Work out the finished part from the listing and answer in its coordinate system (mm). A direction names the side the tool comes from. Coordinates: 2 decimals unless noted, no trailing zeros. Loops run counter-clockwise (first coordinate to the right, second up) from the corner with the lowest first, then second, coordinate; pieces in that order, holes last.
```python
from build123d import *

# Parameters (mm, degrees)
SALIENTE_EXTRUIR1_DEPTH    = 10.8
CORTAR_EXTRUIR1_DEPTH      = 28.076558127
CORTAR_EXTRUIR1_DEPTH_BACK = 28.076558127
CROQUIS4_W                 = 1.025
CROQUIS4_H                 = 17.1
CORTAR_EXTRUIR2_DEPTH      = 33.246404838
CORTAR_EXTRUIR2_DEPTH_BACK = 5.4
CROQUIS5_R                 = 3


with BuildPart() as part:
    # Croquis2 → Saliente-Extruir1 (new, symmetric)
    with BuildSketch(Plane(origin=(0, 0, 0), x_dir=(0, 0, -1), z_dir=(1, 0, 0))):
        with BuildLine():
            Line((11.7, 11.4), (11.7, -21.9))
            Line((11.7, -21.9), (-11.7, -21.9))
            Line((-11.7, -21.9), (-11.7, -12))
            Line((-11.7, -12), (-5.1, -12))
            Line((-5.1, -12), (-5.1, 3))
            ThreePointArc((-5.1, 3), (-3.495742753, 20.791485505), (11.7, 11.4))
        make_face()
    extrude(amount=SALIENTE_EXTRUIR1_DEPTH, both=True)

    # Croquis4 → Cortar-Extruir1 (cut, two sides: drawn at the far end of the back side and taken through both)
    with BuildSketch(Plane.XY.offset(-CORTAR_EXTRUIR1_DEPTH_BACK)):
        with Locations((-10.2875, 13.35)):
            Rectangle(CROQUIS4_W, CROQUIS4_H)
    extrude(amount=CORTAR_EXTRUIR1_DEPTH + CORTAR_EXTRUIR1_DEPTH_BACK, mode=Mode.SUBTRACT)

    # Croquis5 → Cortar-Extruir2 (cut, two sides: drawn at the far end of the back side and taken through both)
    with BuildSketch(Plane.ZY.offset(9.775).offset(-CORTAR_EXTRUIR2_DEPTH_BACK)):
        with Locations(Location((0, 13.35, 0), (0, 0, 90))):
            Circle(CROQUIS5_R)
    extrude(amount=CORTAR_EXTRUIR2_DEPTH + CORTAR_EXTRUIR2_DEPTH_BACK, mode=Mode.SUBTRACT)


solid = part.part
```
1. A cutting plane is placed at B-B, the plane y = 13.35. Give the vertices of the cut face in (x, z) (3 decimals), then the cut area to 3 significant figures.
2. A cutting plane is placed at D-D, the plane y = -5. Give the vertices of the cut face in (x, z), then the cut area to 3 significant figures.
3. A cutting plane is placed at C-C, the plane x = 7.75. Give the vertices of the cut face in (y, z).
4. For faces 5 (the cylindrical face through (0.151, 20.654, 3.761)), 6 (the flat face through (-9.775, 13, -4)), 7 (the flat face through (0, -12, 8)), determine the directions among +Z, -Z, +X, -X, +Y, -Y from which every point of the face is accessible in a straight line to the end or side of a thin tool.
5. Straight lines are drawn through the part: probe 1 along X at (y, z) = (16, -0.75) (3 decimals); probe 2 along Z at (x, y) = (-6, 13.35); probe 3 along Z at (x, y) = (-8.25, 15). For each, find the intervals that lie inside material, in ascending order.
6. A cutting plane is placed at A-A, the plane z = -1.2. Give the vertices of the cut face in (x, y) (3 decimals), then the cut area to 3 significant figures.
7. Determine the mould class of faces 1 (the flat face through (0, -5, 5.1)), 2 (the cylindrical face through (-7.037, 10.353, -0.132)), 3 (the flat face through (-10, 4.8, -2)), 4 (the flat face through (-4.375, 13, 0)) for opening direction Z: released by +Z, released by -Z, zero draft, split by the parting line, or undercut.
8. Each of these flat-tipped pins is pushed along its axis until it touches: P1, Ø1.5, axis at x = -4.5, y = 7, coming from the +Z side; P2, Ø5, axis at x = 0.5, y = -7.5, coming from the +Z side; P3, Ø12, axis at x = -2.5, y = -2, coming from the +Z side. Where does it stop, or does it pass through?
Answers below:
1. outline: (-9.775, -11.517) - (10.8, -11.517) - (10.8, 9.117) - (-9.775, 9.117) - (-9.775, 3) - (-4.375, 3) - (-4.375, -3) - (-9.775, -3) - close
1. area: 392 mm2
2. outline: (-10.8, -11.7) - (10.8, -11.7) - (10.8, 5.1) - (-10.8, 5.1) - close
2. area: 363 mm2
3. outline: (-21.9, -11.7) - (11.4, -11.7) arc R10.5 ccw (long way) to (3, 5.1) - (-12, 5.1) - (-12, 11.7) - (-21.9, 11.7) - close
4. face 5: +X, -X
4. face 6: +Z, -Z, -X, +Y
4. face 7: +Z, +X, -X
5. probe 1: x = -4.375 to 10.8
5. probe 2: z = -11.52 to -3, 3 to 9.12
5. probe 3: z = -11.06 to -2.51, 2.51 to 8.66
6. outline: (-10.8, -21.9) - (10.8, -21.9) - (10.8, 21.9) - (-9.775, 21.9) - (-9.775, 16.1) - (-4.375, 16.1) - (-4.375, 10.6) - (-9.775, 10.6) - (-9.775, 4.8) - (-10.8, 4.8) - close
6. area: 899 mm2
7. face 1: released by +Z
7. face 2: undercut
7. face 3: zero draft
7. face 4: undercut
8. P1: stops at z = 8.65
8. P2: stops at z = 5.1
8. P3: stops at z = 6.25
